Verification items for the finished model (mm, model axes). Round coordinates to 2 decimals unless told otherwise and drop trailing zeros. Order: outer loops, then holes, each group sorted by start corner. A loop starts at its lowest first (then second) coordinate and runs counter-clockwise, first axis right, second up. Notation, with made-up numbers: M 72,-2.75 L 94,-2.75 A10 ccw 94,2.25 Z; hole C 17,72 d9. An arc over 180 degrees is marked long. One line per item, written item: value. Start each with the question number.
from build123d import *

# Parameters (mm, degrees)
BOX001_W     = 1370
BOX001_H     = 160
BOX001_DEPTH = 60
BOX_W        = 1380
BOX_H        = 170
BOX_DEPTH    = 60


with BuildPart() as box001:
    # Box001 → Box001 (new body)
    with BuildSketch(Plane(origin=(5, 5, 5), x_dir=(1, 0, 0), z_dir=(0, 0, 1))):
        with Locations((685, 80)):
            Rectangle(BOX001_W, BOX001_H)
    extrude(amount=BOX001_DEPTH)


with BuildPart() as trough:
    # Box → Box (new body)
    with BuildSketch(Plane.XY):
        with Locations((690, 85)):
            Rectangle(BOX_W, BOX_H)
    extrude(amount=BOX_DEPTH)

    # Cut: cut Box001
    add(box001.part, mode=Mode.SUBTRACT)


with BuildPart() as trough_1:
    # Cut placement: moved
    add(trough.part.moved(Location((66, 0, 0))))


solid = trough_1.part
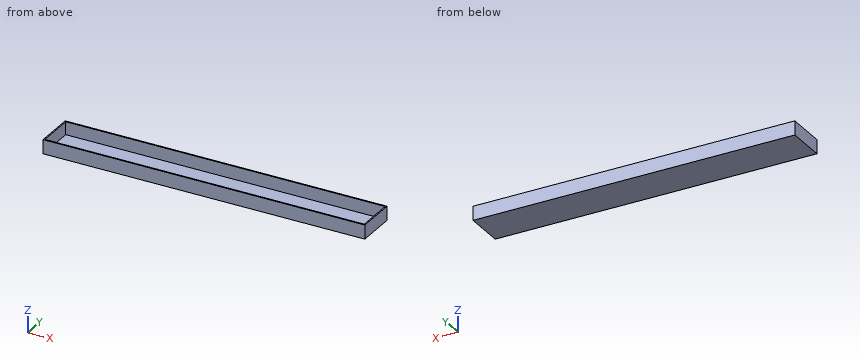
1. Section check C-C (x = 238). Record the cut outline in (y, z), and give its area (3 significant figures).
2. Section check B-B (y = 33.5). Record the cut outline in (x, z).
3. Scan lines: line 1 along X through (y, z) = (50.5, 26); line 2 along Y through (x, z) = (424.5, 46); line 3 along Z through (x, y) = (1371.5, 81.5). Record each from-to range of solid material in increasing order.
4. Depth check by flat-ended pin: pin 1 (10 mm diameter, centred on x = 754, y = 54.5, fed in from +Z). Enter the tip coordinate at first touch or a pass-through.
5. Section check A-A (z = 30). Record the cut outline in (x, y).
Geometry check:
1. outline: M 0,0 L 170,0 L 170,60 L 165,60 L 165,5 L 5,5 L 5,60 L 0,60 Z
1. area: 1,400 mm²
2. outline: M 66,0 L 1446,0 L 1446,60 L 1441,60 L 1441,5 L 71,5 L 71,60 L 66,60 Z
3. line 1: x = 66 to 71, 1441 to 1446
3. line 2: y = 0 to 5, 165 to 170
3. line 3: z = 0 to 5
4. pin 1: stops at z = 5
5. outline: M 66,0 L 1446,0 L 1446,170 L 66,170 Z; hole M 71,5 L 1441,5 L 1441,165 L 71,165 Z
